Verification items for the finished model (mm, model axes). Face numbers are marked on the shaded views. A direction names the side the tool comes from. Give positions to 0.01 mm unless a question says otherwise; leave off trailing zeros. Order: outer loops, then holes, each group sorted by start corner. A loop starts at its lowest first (then second) coordinate and runs counter-clockwise, first axis right, second up. Notation, with made-up numbers: (-38.75, 56) - (-28.75, 56) arc R21 cw to (-28.75, 65) - close; hole circle Ø1 at (41, 84.5). An arc over 180 degrees is marked (long way). Answer as a JSON object with one key per item and string values. Group by question number.
(1) Section check A-A (y = -56). Record the boundary of the cut face in (x, z) (3 decimals), then the cut area to 3 significant figures.
(2) Depth check by flat-ended pin: pin 1 Ø12 at (y, z) = (9, 7.5) entering from +X; pin 2 Ø9 at (x, z) = (149, 0.5) entering from -Y; pin 3 Ø4 at (x, z) = (-10, 2) entering from -Y. Enter the tip coordinate at first touch or a pass-through.
(3) Section check D-D (y = 6). Record the boundary of the cut face in (x, z).
(4) Section check C-C (z = 0). Record the boundary of the cut face in (x, y) (3 decimals).
(5) Access from +Z, -Z, +X, -X, +Y, -Y to the whole of each face (thin tool, end or side, straight path). Record for the marked faces 1, 2 and 3.
(6) Mould release check, pull along Y, two halves, no side actions. Record for the marked faces 4, 5 and 6: +Y half, -Y half, draft (parallel to the pull), parting line (faces both ways), or undercut.
(7) Section check B-B (x = 183). Record the boundary of the cut face in (y, z), then the cut area to 3 significant figures.
(8) Thickness scan on line 1 (Y direction, x = 206, z = 0); line 2 (X direction, y = -4, z = 2); line 3 (Z direction, x = 229.5, y = -49). Record the ranges inside material, lowest first.
```python
from build123d import *

# Parameters (mm, degrees)
BOSS_EXTRUDE1_DEPTH = 50.8
SKETCH2_R           = 19.939
BOSS_EXTRUDE2_DEPTH = 83.82
SKETCH3_W           = 30.48
SKETCH3_H           = 21.336
BOSS_EXTRUDE3_DEPTH = 325.882
SKETCH4_W           = 18.034
SKETCH4_H           = 18.034
BOSS_EXTRUDE4_DEPTH = 20.066
FILLET2_R           = 2.032
SKETCH5_R           = 4.0132
CUT_EXTRUDE1_DEPTH  = 383.778358162
SKETCH6_R           = 9.906
CUT_EXTRUDE2_DEPTH  = 317.5


with BuildPart() as part:
    # Sketch1 → Boss-Extrude1 (new body)
    with BuildSketch(Plane(origin=(0, 0, 0), x_dir=(0, 0, -1), z_dir=(1, 0, 0))):
        with BuildLine():
            Line((-20.955, 0), (-20.955, -61.087))
            Line((-20.955, -61.087), (20.955, -61.087))
            Line((20.955, -61.087), (20.955, 0))
            ThreePointArc((20.955, 0), (0, 20.955), (-20.955, 0))
        make_face()
    extrude(amount=BOSS_EXTRUDE1_DEPTH)

    # Sketch2 → Boss-Extrude2 (add)
    with BuildSketch(Plane(origin=(50.8, 0, 0), x_dir=(0, 0, -1), z_dir=(1, 0, 0))):
        Circle(SKETCH2_R)
    extrude(amount=BOSS_EXTRUDE2_DEPTH)

    # Sketch3 → Boss-Extrude3 (add)
    with BuildSketch(Plane(origin=(50.8, 0, 0), x_dir=(0, 0, -1), z_dir=(1, 0, 0))):
        with BuildLine():
            Line((-15.24, -38.227), (15.24, -38.227))
            ThreePointArc((15.24, -38.227), (0, -22.987), (-15.24, -38.227))
        make_face()
        with Locations((0, -48.895)):
            Rectangle(SKETCH3_W, SKETCH3_H)
    extrude(amount=BOSS_EXTRUDE3_DEPTH)

    # Sketch4 → Boss-Extrude4 (add)
    with BuildSketch(Plane.ZY):
        with Locations((0, -37.211)):
            Rectangle(SKETCH4_W, SKETCH4_H)
    extrude(amount=BOSS_EXTRUDE4_DEPTH)

    # Fillet2
    fillet2_edges = [part.edges().sort_by_distance(p)[0] for p in [
        (-10.033, -28.194, -9.017),
        (-10.033, -46.228, -9.017),
        (-10.033, -46.228, 9.017),
        (-10.033, -28.194, 9.017),
    ]]
    fillet(fillet2_edges, radius=FILLET2_R)

    # Sketch5 → Cut-Extrude1 (cut, through all)
    with BuildSketch(Plane.XY.offset(9.017)):
        with Locations((-11.938, -37.211)):
            Circle(SKETCH5_R)
    extrude(amount=-CUT_EXTRUDE1_DEPTH, mode=Mode.SUBTRACT)

    # Sketch6 → Cut-Extrude2 (cut)
    with BuildSketch(Plane(origin=(376.682, 0, 0), x_dir=(0, 0, -1), z_dir=(1, 0, 0))):
        with Locations((0, -35.687)):
            Circle(SKETCH6_R)
    extrude(amount=-CUT_EXTRUDE2_DEPTH, mode=Mode.SUBTRACT)


solid = part.part
```
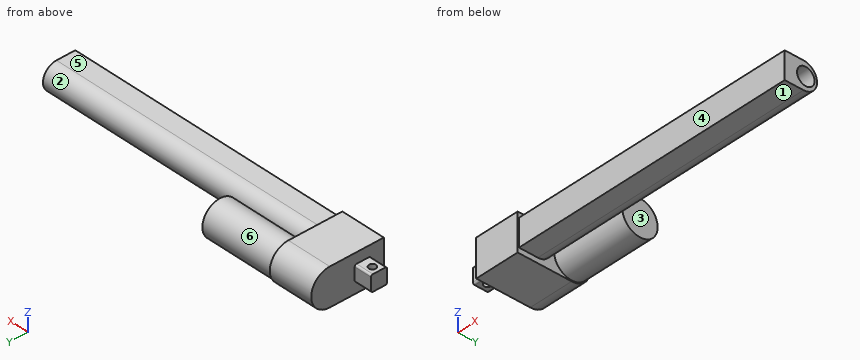
Solutions:
{
 "1": {"outline": "(0, -20.955) - (50.8, -20.955) - (50.8, -15.24) - (376.682, -15.24) - (376.682, 15.24) - (50.8, 15.24) - (50.8, 20.955) - (0, 20.955) - close", "area": "12,100 mm2"},
 "2": {"pin 1": "stops at x = 134.62", "pin 2": "stops at y = -59.56", "pin 3": "stops at y = -46.23"},
 "3": {"outline": "(0, -20.08) - (50.8, -20.08) - (50.8, -19.01) - (134.62, -19.01) - (134.62, 19.01) - (50.8, 19.01) - (50.8, 20.08) - (0, 20.08) - close"},
 "4": {"outline": "(-20.066, -46.228) - (0, -46.228) - (0, -61.087) - (50.8, -61.087) - (50.8, -59.563) - (376.682, -59.563) - (376.682, -45.593) - (59.182, -45.593) - (59.182, -25.781) - (376.682, -25.781) - (376.682, -22.987) - (50.8, -22.987) - (50.8, -19.939) - (134.62, -19.939) - (134.62, 19.939) - (50.8, 19.939) - (50.8, 20.955) - (0, 20.955) - (0, -28.194) - (-20.066, -28.194) - close; hole circle Ø8.026 at (-11.938, -37.211)"},
 "5": {"face 1": "-Z, +X, -Y", "face 2": "+X", "face 3": "+Z, -Z, +X, +Y"},
 "6": {"face 4": "-Y half", "face 5": "draft", "face 6": "undercut"},
 "7": {"outline": "(-59.56, -15.24) - (-38.23, -15.24) arc R15.24 ccw to (-38.23, 15.24) - (-59.56, 15.24) - close; hole circle Ø19.81 at (-35.69, 0)", "area": "707 mm2"},
 "8": {"line 1": "y = -59.56 to -45.59, -25.78 to -22.99", "line 2": "x = 0 to 134.62", "line 3": "z = -15.24 to 15.24"}
}
